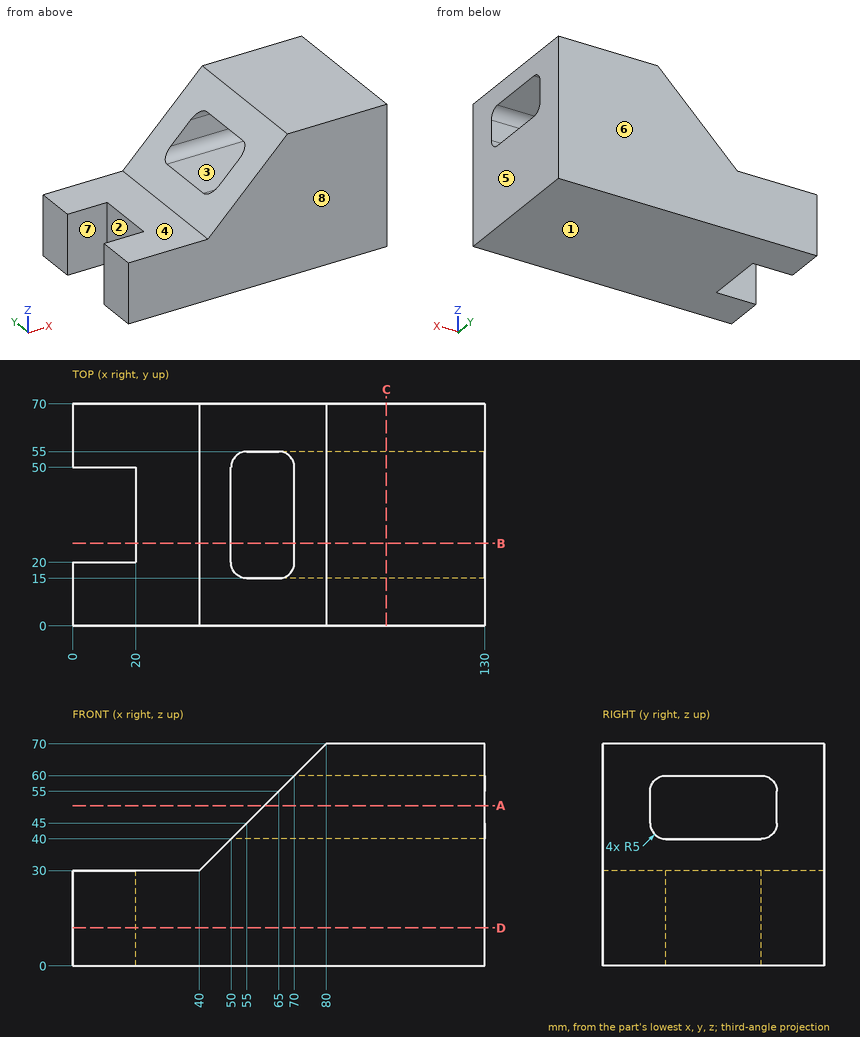
Design review of the part shown in the three views and the two pictorial views. Dimensions are in mm from the part's minimum x, y and z. A direction names the side the tool comes from. Round coordinates to 2 decimals unless told otherwise and drop trailing zeros. Loops run counter-clockwise (first coordinate to the right, second up) from the corner with the lowest first, then second, coordinate; pieces in that order, holes last. Notation, with made-up numbers: (8.25, -38.75) - (64.25, -38.75) arc R30 ccw to (64.25, -8.75) - close; hole circle Ø4 at (67, -37.75). An arc over 180 degrees is marked (long way). Answer as CSV lines item,"result".
(1) Mouldability with a two-part tool opening along Y and no side actions: class the marked faces 5, 6, 7 and 8 as +Y half, -Y half, draft (parallel to the pull), parting line (faces both ways), or undercut.
Checked values:
face 5,"draft"
face 6,"+Y half"
face 7,"undercut"
face 8,"-Y half"
(2) Insertion check: P1, Ø8, axis at x = 47.5, y = 27.5, coming from the -Z side; P2, Ø12, axis at x = 14, y = 52, coming from the +Z side. Each pin has a flat end and moves straight along its axis. Give the tip position at first contact, or say it passes through.
Checked values:
P1,"stops at z = 0"
P2,"stops at z = 30"
(3) Consider section C-C on x = 99. Give the boundary of the cut face in (y, z).
Checked values:
outline,"(0, 0) - (70, 0) - (70, 70) - (0, 70) - close; hole (15, 45) arc R5 ccw to (20, 40) - (50, 40) arc R5 ccw to (55, 45) - (55, 55) arc R5 ccw to (50, 60) - (20, 60) arc R5 ccw to (15, 55) - close"
(4) Wall thickness on line 1 (Y direction, x = 7, z = 6.5); line 2 (Y direction, x = 118, z = 54); line 3 (X direction, y = 19, z = 35): over which ranges is each line inside the solid? List them lowest first.
Checked values:
line 1,"y = 0 to 20, 50 to 70"
line 2,"y = 0 to 15, 55 to 70"
line 3,"x = 45 to 130"
(5) Consider section D-D on z = 12. Give the boundary of the cut face in (x, y), then the cut area to 3 significant figures.
Checked values:
outline,"(0, 0) - (130, 0) - (130, 70) - (0, 70) - (0, 50) - (20, 50) - (20, 20) - (0, 20) - close"
area,"8,500 mm2"
(6) Consider section A-A on z = 50.5. Give the boundary of the cut face in (x, y), then the cut area to 4 significant figures.
Checked values:
outline,"(60.5, 0) - (130, 0) - (130, 15) - (60.5, 15) - close; (60.5, 55) - (130, 55) - (130, 70) - (60.5, 70) - close"
area,"2,085 mm2"
(7) Consider section B-B on y = 26. Give the boundary of the cut face in (x, z), then the cut area to 3 significant figures.
Checked values:
outline,"(20, 0) - (130, 0) - (130, 40) - (50, 40) - (40, 30) - (20, 30) - close; (70, 60) - (130, 60) - (130, 70) - (80, 70) - close"
area,"4,700 mm2"
(8) Tool access review of the marked faces 1, 2, 3 and 4: name each direction out of +Z, -Z, +X, -X, +Y, -Y from which nothing blocks a thin tool from reaching the whole face with its end or side.
Checked values:
face 1,"-Z, +X, -X, +Y, -Y"
face 2,"+Z, -Z, -X"
face 3,"+X, -X"
face 4,"+Z, -X, +Y, -Y"
